Could you check a few things on this drawing? It's one solid part, dimensions in mm from its lowest x, y, z. A direction names the side the tool comes from. Round coordinates to 2 decimals unless told otherwise and drop trailing zeros. Order: outer loops, then holes, each group sorted by start corner. A loop starts at its lowest first (then second) coordinate and runs counter-clockwise, first axis right, second up.
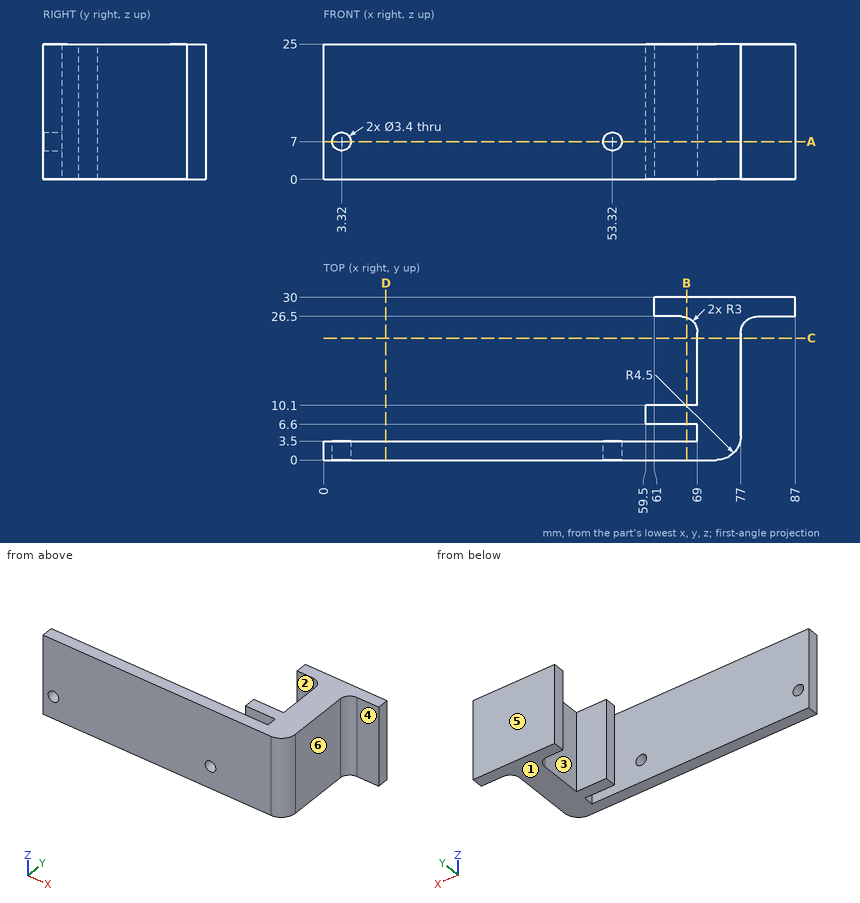
(1) I want a section at D-D, the plane x = 11.5. List the corners of the cut face in (y, z) for me, plus the area to 3 significant figures.
(2) I want a section at B-B, the plane x = 67. List the corners of the cut face in (y, z) for me, plus the area to 3 significant figures.
(3) If we mould it in two halves opening along Y, with no side actions, what happens to the marked faces 3, 4, 5 and 6? For each: pulls with the +Y half, pulls with the -Y half, needs draft (parallel to the pull), parting line crosses it, or undercut.
(4) I want a section at A-A, the plane z = 7. List the corners of the cut face in (x, y) for me.
(5) On a 3-axis mill with a long thin cutter (end or side, diameter ignored), from which of +Z, -Z, +X, -X, +Y, -Y can I reach the whole of each face in a straight line? I mean the marked faces 1 and 2. Say none if no direction works.
(6) I want a section at C-C, the plane y = 22.5. List the corners of the cut face in (x, z) for me.
(7) Please list where these lines run through material, in increasing order: probe 1 along X at (y, z) = (1.25, 7); probe 2 along X at (y, z) = (0.9, 7); probe 3 along Y at (x, z) = (67, 17).
(8) I'm going to push flat-ended pins straight in: pin 1 Ø4 at (y, z) = (16.5, 7.5) entering from -X; pin 2 Ø12 at (x, z) = (25, 10) entering from -Y; pin 3 Ø4 at (x, z) = (53.32, 7) entering from +Y; pin 4 Ø1.8 at (y, z) = (28, 15.5) entering from -X. Where does each tip first touch, or does it pass through?
Ans:
1. outline: (0, 0) - (3.5, 0) - (3.5, 25) - (0, 25) - close
1. area: 87.5 mm2
2. outline: (0, 0) - (3.5, 0) - (3.5, 25) - (0, 25) - close; (6.6, 0) - (10.1, 0) - (10.1, 25) - (6.6, 25) - close; (26.33, 0) - (30, 0) - (30, 25) - (26.33, 25) - close
2. area: 267 mm2
3. face 3: undercut
3. face 4: pulls with the -Y half
3. face 5: pulls with the +Y half
3. face 6: needs draft
4. outline: (0, 0) - (1.62, 0) - (1.62, 3.5) - (0, 3.5) - close; (5.02, 0) - (51.62, 0) - (51.62, 3.5) - (5.02, 3.5) - close; (55.02, 0) - (72.5, 0) arc R4.5 ccw to (77, 4.5) - (77, 23.5) arc R3 cw to (80, 26.5) - (87, 26.5) - (87, 30) - (61, 30) - (61, 26.5) - (66, 26.5) arc R3 cw to (69, 23.5) - (69, 10.1) - (59.5, 10.1) - (59.5, 6.6) - (69, 6.6) - (69, 3.5) - (55.02, 3.5) - close
5. face 1: -Z, +X, -X, +Y, -Y
5. face 2: +Z, -Z, -X
6. outline: (69, 0) - (77, 0) - (77, 25) - (69, 25) - close
7. probe 1: x = 0 to 1.62, 5.02 to 51.62, 55.02 to 75.61
7. probe 2: x = 0 to 1.62, 5.02 to 51.62, 55.02 to 75.2
7. probe 3: y = 0 to 3.5, 6.6 to 10.1, 26.33 to 30
8. pin 1: stops at x = 69
8. pin 2: stops at y = 0
8. pin 3: stops at y = 3.5
8. pin 4: stops at x = 61
